Drawing for the job (mm, zero at the part's lowest x, y, z). A direction names the side the tool comes from. Coordinates: 2 decimals unless noted, no trailing zeros. Loops run counter-clockwise (first coordinate to the right, second up) from the corner with the lowest first, then second, coordinate; pieces in that order, holes last. Notation, with made-up numbers: (57, -10) - (87, -10) arc R34 cw to (87, 20) - close; hole circle Ø2 at (85, -27.75). An arc over 180 degrees is marked (long way). Put each result on its own line as item: value.
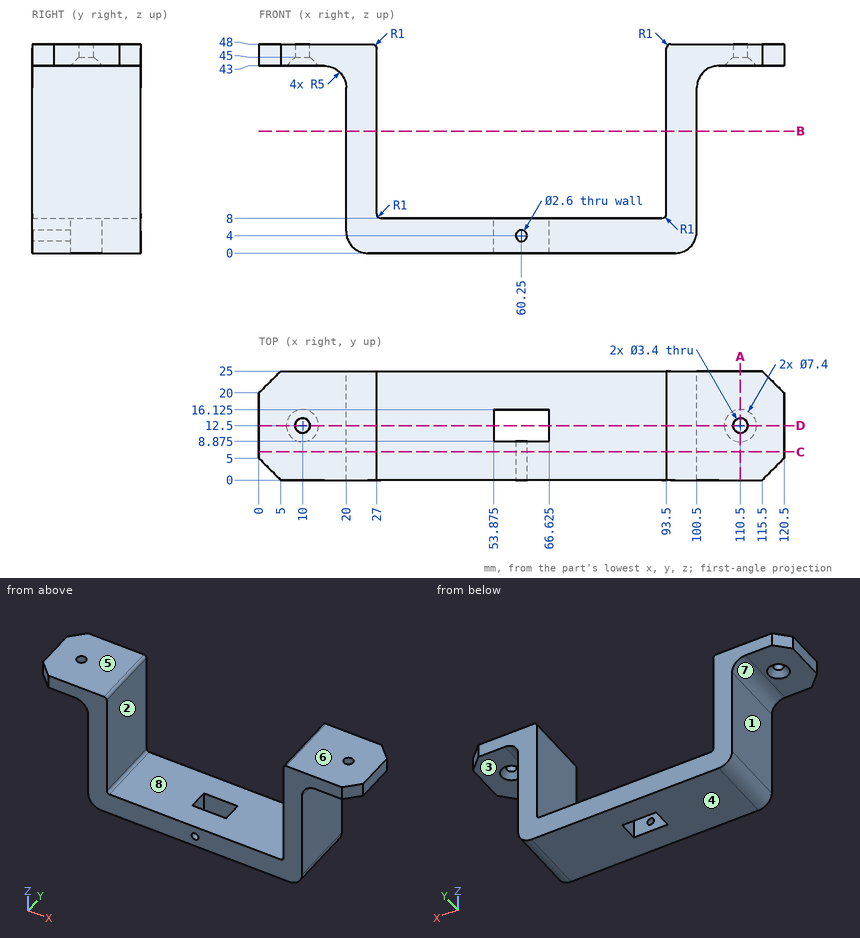
Q1. Tool access for the marked faces 1, 2, 3, 4 and 5: list every direction of +Z, -Z, +X, -X, +Y, -Y with a clear straight run to the whole face (end or side of a thin tool).
Determined:
face 1: -Z, -X, +Y, -Y
face 2: +Z, +Y, -Y
face 3: -Z, +X, +Y, -Y
face 4: -Z, +X, -X, +Y, -Y
face 5: +Z, +X, -X, +Y, -Y
Q2. Slice it at B-B, the plane z = 28. Give the cut face in (x, y), then the cut area to 3 significant figures.
Determined:
outline: (20, 0) - (27, 0) - (27, 25) - (20, 25) - close; (93.5, 0) - (100.5, 0) - (100.5, 25) - (93.5, 25) - close
area: 350 mm2
Q3. Slice it at C-C, the plane y = 6.5. Give the cut face in (x, z), then the cut area to 3 significant figures.
Determined:
outline: (0, 43) - (15, 43) arc R5 cw to (20, 38) - (20, 5) arc R5 ccw to (25, 0) - (95.5, 0) arc R5 ccw to (100.5, 5) - (100.5, 38) arc R5 cw to (105.5, 43) - (120.5, 43) - (120.5, 48) - (94.5, 48) arc R1 ccw to (93.5, 47) - (93.5, 9) arc R1 cw to (92.5, 8) - (28, 8) arc R1 cw to (27, 9) - (27, 47) arc R1 ccw to (26, 48) - (0, 48) - close; hole circle Ø2.6 at (60.25, 4)
area: 1,400 mm2
Q4. Mould opens along X. For the marked faces 6, 7 and 8 say: +X half, -X half, draft (parallel to the pull), parting line (faces both ways), or undercut.
Determined:
face 6: draft
face 7: -X half
face 8: undercut
Q5. Pin check, flat tips, straight feed: pin 1 Ø12.5 at (y, z) = (6.5, 32.5) entering from -X; pin 2 Ø2 at (y, z) = (12.5, 4.5) entering from -X; pin 3 Ø2 at (x, z) = (60.25, 4) entering from -Y (3 decimals); pin 4 Ø4 at (x, z) = (52.5, 11) entering from -Y. Stop position of each tip, or through.
Determined:
pin 1: x = 19.94
pin 2: x = 20
pin 3: y = 16.125
pin 4: through
Q6. Slice it at A-A, the plane x = 110.5. Give the cut face in (y, z).
Determined:
outline: (0, 43) - (8.8, 43) - (10.8, 45) - (10.8, 48) - (0, 48) - close; (14.2, 45) - (16.2, 43) - (25, 43) - (25, 48) - (14.2, 48) - close
Q7. Wall check: L1, parallel to X at y = 12.5, z = 47.05; L2, parallel to X at y = 3.75, z = 10; L3, parallel to Y at x = 110.5, z = 46.8. Give the ranges that are in metal, low to high. Write a range as from..to.
Determined:
L1: 0..8.3, 11.7..27, 93.5..108.8, 112.2..120.5
L2: 20..27, 93.5..100.5
L3: 0..10.8, 14.2..25
Q8. Slice it at D-D, the plane y = 12.5. State how many separate pieces and enclosed holes the cut face has, then the cut area to 3 significant figures.
Determined:
separate pieces: 4
enclosed holes: 0
area: 1,260 mm2
